Design review of the part built by this model. Coordinates are the model's own, in mm. A direction names the side the tool comes from. Give positions to 0.01 mm unless a question says otherwise; leave off trailing zeros. Loops run counter-clockwise (first coordinate to the right, second up) from the corner with the lowest first, then second, coordinate; pieces in that order, holes last. Notation, with made-up numbers: M 86.25,-14 L 104.25,-14 A21 ccw 104.25,-2 Z; hole C 72.25,78 d2. An arc over 180 degrees is marked long. Answer as CSV lines item,"result".
```python
from build123d import *

# Parameters (mm, degrees)
SKETCH1_R           = 1
BOSS_EXTRUDE1_DEPTH = 5.3
SKETCH2_W           = 1
SKETCH2_H           = 7.632118098
CUT_EXTRUDE1_DEPTH  = 24.262242696
BOSS_EXTRUDE2_DEPTH = 6
SKETCH5_R           = 1.5
CUT_EXTRUDE2_DEPTH  = 14.937332122
CUT_EXTRUDE3_START  = -3
CUT_EXTRUDE3_DEPTH  = 3


# Read off the part's stored shape, not the designer's step: Cut-Extrude3
with BuildPart() as part:
    # Sketch1 → Boss-Extrude1 (new body)
    with BuildSketch(Plane.XY):
        with BuildLine():
            Line((-7.5, 0), (7.5, 0))
            Line((7.5, 0), (10, 2.5))
            Line((10, 2.5), (10, 10.632118098))
            Line((10, 10.632118098), (6.075, 10.632118098))
            Line((6.075, 10.632118098), (6.075, 7.547815402))
            ThreePointArc((6.075, 7.547815402), (4.848419821, 4.342215517), (1.689491671, 3))
            Line((1.689491671, 3), (-1.689458819, 3))
            ThreePointArc((-1.689458819, 3), (-4.736103523, 4.229921298), (-6.075, 7.230272374))
            Line((-6.075, 7.230272374), (-6.075, 10.632118098))
            Line((-6.075, 10.632118098), (-10, 10.632118098))
            Line((-10, 10.632118098), (-10, 2.5))
            Line((-10, 2.5), (-7.5, 0))
        make_face()
        with Locations((-8, 7.5)):
            Circle(SKETCH1_R, mode=Mode.SUBTRACT)
        with Locations((8, 7.5)):
            Circle(SKETCH1_R, mode=Mode.SUBTRACT)
    extrude(amount=BOSS_EXTRUDE1_DEPTH)

    # Sketch2 → Cut-Extrude1 (cut, through all)
    with BuildSketch(Plane(origin=(10, 0, 0), x_dir=(0, 0, -1), z_dir=(1, 0, 0))):
        with Locations((-2.65, 6.816059049)):
            Rectangle(SKETCH2_W, SKETCH2_H)
    extrude(amount=-CUT_EXTRUDE1_DEPTH, mode=Mode.SUBTRACT)

    # Sketch3 → Boss-Extrude2 (add)
    with BuildSketch(Plane(origin=(0, 0, 0), x_dir=(-1, 0, 0), z_dir=(0, 0, -1))):
        Polygon((10, 2.5), (10, 3), (1.689458819, 3), (-1.689491671, 3), (-10, 3), (-10, 2.5), (-7.5, 0), (7.5, 0), align=None)
    extrude(amount=BOSS_EXTRUDE2_DEPTH)

    # Sketch5 → Cut-Extrude2 (cut, through all)
    with BuildSketch(Plane(origin=(0, 3, 0), x_dir=(1, 0, 0), z_dir=(0, 1, 0))):
        with Locations(Location((-5, 3, 0), (0, 0, 270))):
            Circle(SKETCH5_R)
        with Locations(Location((5, 3, 0), (0, 0, 90))):
            Circle(SKETCH5_R)
    extrude(amount=-CUT_EXTRUDE2_DEPTH, mode=Mode.SUBTRACT)

    # Cut-Extrude3 outline → Cut-Extrude3 (cut)
    with BuildSketch(Plane(origin=(0, 3, 0), x_dir=(1, 0, 0), z_dir=(0, 1, 0)).offset(CUT_EXTRUDE3_START)):
        with BuildLine():
            ThreePointArc((-6.14052533, 5.774743587), (-5.581278436, 5.94314719), (-5, 6))
            Line((-5, 6), (-10, 6))
            Line((-10, 6), (-10, 0.031065848))
            ThreePointArc((-10, 0.031065848), (-8.941597101, 3.488399471), (-6.14052533, 5.774743587))
        make_face()
        with BuildLine():
            ThreePointArc((6.14052533, 5.774743587), (8.941597101, 3.488399471), (10, 0.031065848))
            Line((10, 0.031065848), (10, 6))
            Line((10, 6), (5, 6))
            ThreePointArc((5, 6), (5.581278436, 5.94314719), (6.14052533, 5.774743587))
        make_face()
    extrude(amount=CUT_EXTRUDE3_DEPTH, mode=Mode.SUBTRACT)


solid = part.part
```
1. We need section A-A, the plane z = 3.5. Write out the cut boundary in (x, y) (1 decimal).
Answer block:
outline,"M -10,2.5 L -7.5,0 L 7.5,0 L 10,2.5 L 10,10.6 L 6.1,10.6 L 6.1,7.5 A4.4 cw 1.7,3 L -1.7,3 A4.4 cw -6.1,7.2 L -6.1,10.6 L -10,10.6 Z; hole C -8,7.5 d2; hole C 8,7.5 d2"
2. To check wall thickness, follow L1, parallel to X at y = 7.5, z = 1 (3 decimals); L2, parallel to X at y = 1.95, z = -3; L3, parallel to Z at x = 5, y = 1.4. State the ranges of each line that lie inside material, in increasing order. Write a range as [from, to].
Answer block:
L1,"[-10, -9], [-7, -6.075], [6.076, 7], [9, 10]"
L2,"[-9.24, -6.5], [-3.5, 3.5], [6.5, 9.24]"
L3,"[-6, -4.5], [-1.5, 5.3]"
3. For P1, Ø2.5, axis at x = -8, y = 7.5, coming from the -Z side; P2, Ø1, axis at x = 4.5, z = -4, coming from the -Y side; P3, Ø1.5, axis at y = 1.5, z = 0.5, coming from the +X side; P4, Ø5.5, axis at x = -2, z = -1.5, coming from the +Y side, all flat-tipped, find the tip position at first contact; note any pin that passes through.
Answer block:
P1,"z = 0"
P2,"y = 0"
P3,"x = 9.75"
P4,"y = 3.86"
4. We need section D-D, the plane z = -3. Write out the cut boundary in (x, y).
Answer block:
outline,"M -9.24,1.74 L -7.5,0 L -6.5,0 L -6.5,3 L -9.24,3 Z; M -3.5,0 L 3.5,0 L 3.5,3 L -3.5,3 Z; M 6.5,0 L 7.5,0 L 9.24,1.74 L 9.24,3 L 6.5,3 Z"
5. We need section C-C, the plane y = 2.75. Write out the cut boundary in (x, z).
Answer block:
outline,"M -10,-0.03 A6.23 ccw -6.14,-5.77 A3 ccw -5,-6 L 5,-6 A3 ccw 6.14,-5.77 A6.23 ccw 10,-0.03 L 10,5.3 L -10,5.3 Z; hole C -5,-3 d3; hole C 5,-3 d3"
6. The part is to be moulded in two halves that separate along X. For faces 4 (the flat face through (-8, 6, 3.15)), 5 (the flat face through (-8.7, 1.2, 0.2)), 6 (the flat face through (8.8, 1.3, 0.2)), 7 (the flat face through (6.075, 9, 1)), say which applies: pulls with the +X half, pulls with the -X half, needs draft (parallel to the pull), parting line crosses it, or undercut.
Answer block:
face 4,"needs draft"
face 5,"pulls with the -X half"
face 6,"pulls with the +X half"
face 7,"undercut"
7. For faces 1 (the flat face through (6.075, 9, 4)), 2 (the cylindrical face through (7.87, 8.49, 1.06)), 3 (the flat face through (-8, 6, 0)), list the 3-axis set-ups (+Z, -Z, +X, -X, +Y, -Y) from which the entire face can be reached by the end or side of a thin tool; tool diameter is ignored.
Answer block:
face 1,"+Z, -Z, +Y"
face 2,"+Z, -Z"
face 3,"-Z, +X, -X, +Y"
8. We need section B-B, the plane y = 9. Write out the cut boundary in (x, z) (3 decimals), plus the area to 3 significant figures.
Answer block:
outline,"M -10,0 L -6.075,0 L -6.075,2.15 L -10,2.15 Z; M -10,3.15 L -6.075,3.15 L -6.075,5.3 L -10,5.3 Z; M 6.075,0 L 10,0 L 10,2.15 L 6.075,2.15 Z; M 6.075,3.15 L 10,3.15 L 10,5.3 L 6.075,5.3 Z"
area,"33.8 mm²"
